Could you check a few things on this model? Use its own coordinates, in mm. A direction names the side the tool comes from. Coordinates: 2 decimals unless noted, no trailing zeros. Write each loop counter-clockwise with the first axis right and the second up, starting at its lowest first coordinate (ties: lowest second). Pieces come first, ordered by that corner, then holes.
Item 1: For P1, Ø2, axis at x = 44.5, z = -8, coming from the +Y side; P2, Ø12, axis at y = 0, z = 0, coming from the -X side; P3, Ø1.5, axis at x = 60, z = 5, coming from the +Y side, each with a flat end and sliding along its axis, tell me the tip position at first contact or that it passes through.
Item 2: I want a section at D-D on x = 25. Please give me the cut outline in (y, z).
Item 3: I want a section at B-B on z = 0. Please give me the cut outline in (x, y), then the cut area to 3 significant figures.
Item 4: I want a section at C-C on x = 61.5. Please give me the cut outline in (y, z).
Item 5: If I drill on probe 1 along Y at (x, z) = (80.5, 0); probe 2 along Y at (x, z) = (30, 0); probe 3 along Z at (x, y) = (58.5, 0.75), over which ranges is the centre line in solid material (lowest first)?
Item 6: Which directions (+Z, -Z, +X, -X, +Y, -Y) give clear straight access to the entire face, cutting with the end or side of a thin tool? Please do faces 1 (the cylindrical face through (86, 2, 0)), 2 (the cylindrical face through (31, 0, -10)), 3 (the flat face through (5, -11.05, 0)).
Item 7: I want a section at A-A on y = 0. Please give me the cut outline in (x, z), then the cut area to 3 significant figures.
from build123d import *

# Parameters (mm, degrees)
ESQUISSE2_W             = 10
ESQUISSE2_H             = 22.1
ENL_V_MAT_EXTRU_1_DEPTH = 15


with BuildPart() as part:
    # Esquisse1 → Révolution1 (revolve)
    with BuildSketch(Plane.XY, mode=Mode.PRIVATE) as r_volution1_sk:
        with BuildLine():
            Line((56.618802154, 2), (52, 10))
            Line((52, 10), (0, 10))
            Line((0, 10), (0, 12.5))
            Line((0, 12.5), (92, 12.5))
            Line((92, 12.5), (113.418113853, 10.248865523))
            ThreePointArc((113.418113853, 10.248865523), (115.972579302, 8.947300367), (117, 6.270777941))
            Line((117, 6.270777941), (117, 2))
            Line((117, 2), (56.618802154, 2))
        make_face()
    revolve(r_volution1_sk.sketch.rotate(Axis((0, 0, 0), (1, 0, 0)), 90), axis=Axis((0, 0, 0), (1, 0, 0)))  # turned: the seam where the file's is

    # Esquisse2 → Enlèv. mat.-Extru.1 (cut, symmetric)
    with BuildSketch(Plane.XY):
        with Locations((5, 0)):
            Rectangle(ESQUISSE2_W, ESQUISSE2_H)
    extrude(amount=ENL_V_MAT_EXTRU_1_DEPTH, both=True, mode=Mode.SUBTRACT)


solid = part.part
Response values:
1. P1: stops at y = 10.36
1. P2: stops at x = 54.31
1. P3: stops at y = 11.76
2. outline: circle Ø25 at (0, 0); hole circle Ø20 at (0, 0)
3. outline: (0, -12.5) - (92, -12.5) - (113.42, -10.25) arc R4 ccw to (117, -6.27) - (117, -2) - (56.62, -2) - (52, -10) - (10, -10) - (10, -11.05) - (0, -11.05) - close; (0, 11.05) - (10, 11.05) - (10, 10) - (52, 10) - (56.62, 2) - (117, 2) - (117, 6.27) arc R4 ccw to (113.42, 10.25) - (92, 12.5) - (0, 12.5) - close
3. area: 1,500 mm2
4. outline: circle Ø25 at (0, 0); hole circle Ø4 at (0, 0)
5. probe 1: y = -12.5 to -2, 2 to 12.5
5. probe 2: y = -12.5 to -10, 10 to 12.5
5. probe 3: z = -12.48 to -1.85, 1.85 to 12.48
6. face 1: +X, -X
6. face 2: -X
6. face 3: +Z, -Z, -X
7. outline: (10, -12.5) - (92, -12.5) - (113.42, -10.25) arc R4 ccw to (117, -6.27) - (117, -2) - (56.62, -2) - (52, -10) - (10, -10) - close; (10, 10) - (52, 10) - (56.62, 2) - (117, 2) - (117, 6.27) arc R4 ccw to (113.42, 10.25) - (92, 12.5) - (10, 12.5) - close
7. area: 1,470 mm2
